```python
from build123d import *

# Parameters (mm, degrees)
SKETCH1_W           = 15
SKETCH1_H           = 5.2
SKETCH1_W_2         = 5.2
SKETCH1_H_2         = 30
SKETCH1_H_3         = 15
BOSS_EXTRUDE1_DEPTH = 5


with BuildPart() as part:
    # Sketch1 → Boss-Extrude1 (new body)
    with BuildSketch(Plane(origin=(0, 0, 0), x_dir=(1, 0, 0), z_dir=(0, 1, 0))):
        Polygon((92.514530464, -147.019914311), (92.514530464, 52.980085689), (-80.485469536, 52.980085689), (-130.485469536, 27.980085689), (-213.485469536, 27.980085689), (-213.485469536, -122.019914311), (-130.485469536, -122.019914311), (-80.485469536, -147.019914311), align=None)
        with Locations((75.014530464, 47.380085689)):
            Rectangle(SKETCH1_W, SKETCH1_H, mode=Mode.SUBTRACT)
        with Locations((75.014530464, -141.419914311)):
            Rectangle(SKETCH1_W, SKETCH1_H, mode=Mode.SUBTRACT)
        with Locations((86.914530464, -0.019914311)):
            Rectangle(SKETCH1_W_2, SKETCH1_H_2, mode=Mode.SUBTRACT)
        with Locations((86.914530464, -47.019914311)):
            Rectangle(SKETCH1_W_2, SKETCH1_H_2, mode=Mode.SUBTRACT)
        with Locations((86.914530464, -94.019914311)):
            Rectangle(SKETCH1_W_2, SKETCH1_H_2, mode=Mode.SUBTRACT)
        with Locations((-9.785469536, 47.373767599)):
            Rectangle(SKETCH1_W, SKETCH1_H, mode=Mode.SUBTRACT)
        with Locations((-47.985469536, 47.373767599)):
            Rectangle(SKETCH1_W, SKETCH1_H, mode=Mode.SUBTRACT)
        with Locations((-148.485469536, 22.380085689)):
            Rectangle(SKETCH1_W, SKETCH1_H, mode=Mode.SUBTRACT)
        with Locations((-190.985469536, 22.380085689)):
            Rectangle(SKETCH1_W, SKETCH1_H, mode=Mode.SUBTRACT)
        with Locations((-207.885469536, -3.519914311)):
            Rectangle(SKETCH1_W_2, SKETCH1_H_3, mode=Mode.SUBTRACT)
        with Locations((-207.885469536, -47.019914311)):
            Rectangle(SKETCH1_W_2, SKETCH1_H_2, mode=Mode.SUBTRACT)
        with Locations((-207.885469536, -90.519914311)):
            Rectangle(SKETCH1_W_2, SKETCH1_H_3, mode=Mode.SUBTRACT)
        with Locations((-48.86060515, -141.420106162)):
            Rectangle(SKETCH1_W, SKETCH1_H, mode=Mode.SUBTRACT)
        with Locations((-148.485469536, -116.419914311)):
            Rectangle(SKETCH1_W, SKETCH1_H, mode=Mode.SUBTRACT)
        with Locations((-190.985469536, -116.419914311)):
            Rectangle(SKETCH1_W, SKETCH1_H, mode=Mode.SUBTRACT)
        with Locations((28.414530464, 47.380085689)):
            Rectangle(SKETCH1_W, SKETCH1_H, mode=Mode.SUBTRACT)
        with Locations((28.414530464, -141.419914311)):
            Rectangle(SKETCH1_W, SKETCH1_H, mode=Mode.SUBTRACT)
        with Locations((-9.785469536, -141.413596222)):
            Rectangle(SKETCH1_W, SKETCH1_H, mode=Mode.SUBTRACT)
        Polygon((-110.963133782, 28.573374858), (-113.288285266, 33.223677824), (-126.704693131, 26.515473891), (-124.379541647, 21.865170925), align=None, mode=Mode.SUBTRACT)
        Polygon((-86.455469536, 46.640085689), (-84.130318052, 41.989782723), (-97.546725917, 35.28157879), (-99.871877401, 39.931881756), align=None, mode=Mode.SUBTRACT)
        Polygon((-99.871877401, -133.971710379), (-86.455469536, -140.679914311), (-84.130318052, -136.029611345), (-97.546725917, -129.321407413), align=None, mode=Mode.SUBTRACT)
        Polygon((-124.379541647, -115.904999548), (-110.963133782, -122.61320348), (-113.288285266, -127.263506446), (-126.704693131, -120.555302514), align=None, mode=Mode.SUBTRACT)
    extrude(amount=BOSS_EXTRUDE1_DEPTH)


solid = part.part
```
Source: CAD feature listing. Evaluate the final solid. Frame: model axes, mm. A direction names the side the tool comes from. Round coordinates to 2 decimals unless told otherwise and drop trailing zeros. Write each loop counter-clockwise with the first axis right and the second up, starting at its lowest first coordinate (ties: lowest second). Pieces come first, ordered by that corner, then holes. Notation, with made-up numbers: M 80.5,-7.5 L 103.5,-7.5 A24 cw 103.5,21.5 Z; hole C 2,47.5 d10. An arc over 180 degrees is marked long. Answer as a JSON object with one key per item and string values. Group by question number.
(1) Section query D-D on x = -137. Output: boundary loops of the cut face in (y, z), then the cut area to 3 significant figures.
(2) Ray query, line 1 (X direction, y = 2.8, z = 33.5); line 2 (Z direction, x = -52.5, y = 3.65); line 3 (Z direction, x = -185, y = 1.45). Return the intervals inside material, ascending. Write a range as [from, to].
(3) Reachability of faces 1 (the flat face through (-63, 0, 46)), 2 (the flat face through (-119.9, 2.46, -29.92)) from +Z, -Z, +X, -X, +Y, -Y: full face, straight path, thin tool, end or side. Return the list, or none.
(4) Section query B-B on x = -52. Output: boundary loops of the cut face in (y, z), then the cut area to 3 significant figures.
(5) Section query C-C on y = 3.45. State how many separate pieces and enclosed holes the cut face has, then the cut area to 3 significant figures.
(6) Mould query, pull axis X, two halves, no side actions, for faces 3 (the flat face through (-105.835, 2.465, 134.345)), 4 (the flat face through (-63, 5, 46)), 5 (the flat face through (-119.903, 2.465, 123.956)), 6 (the flat face through (-93.26, 2.46, -43.24)). Classes: +X half, -X half, draft (parallel to the pull), parting line (faces both ways), or undercut.
(7) First-contact query: pin 1 (1.5 mm diameter, centred on x = -207, y = 3.5, fed in from -Z). Flat tip, straight axial feed; report the tip coordinate or a pass-through.
(8) Section query A-A on z = 44.5. Output: boundary loops of the cut face in (x, y), then the cut area to 3 significant figures.
Computed values:
{
 "1": {"outline": "M 0,-27.98 L 5,-27.98 L 5,122.02 L 0,122.02 Z", "area": "750 mm^2"},
 "2": {"line 1": "[-213.49, -210.49], [-205.29, 84.31], [89.51, 92.51]", "line 2": "[-52.98, -49.97], [-44.77, 138.82], [144.02, 147.02]", "line 3": "[-27.98, -24.98], [-19.78, 113.82], [119.02, 122.02]"},
 "3": {"face 1": "+Z, -Z, +X, -X, -Y", "face 2": "+Y, -Y"},
 "4": {"outline": "M 0,-52.98 L 5,-52.98 L 5,-49.97 L 0,-49.97 Z; M 0,-44.77 L 5,-44.77 L 5,138.82 L 0,138.82 Z; M 0,144.02 L 5,144.02 L 5,147.02 L 0,147.02 Z", "area": "948 mm^2"},
 "5": {"separate pieces": "1", "enclosed holes": "22", "area": "53,800 mm^2"},
 "6": {"face 3": "-X half", "face 4": "draft", "face 5": "undercut", "face 6": "undercut"},
 "7": {"pin 1": "z = -27.98"},
 "8": {"outline": "M -213.49,0 L -210.49,0 L -210.49,5 L -213.49,5 Z; M -205.29,0 L 84.31,0 L 84.31,5 L -205.29,5 Z; M 89.51,0 L 92.51,0 L 92.51,5 L 89.51,5 Z", "area": "1,480 mm^2"}
}
